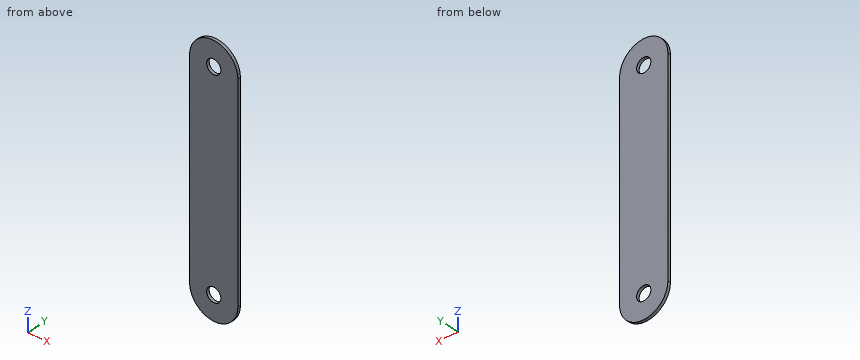
Solid Edge part; units mm, degrees
sketch "Sketch1" plane through (0, 0, 0) normal (0, -1, 0) x (1, 0, 0)
  circle A0 centre (0, 36.395) radius 2.5
  line L0 (-8.5, -36.755) -> (-8.5, 36.395)
  line L1 (8.5, 36.395) -> (8.5, -36.755)
  arc A1 (-8.5, 36.395) -> (8.5, 36.395) centre (0, 36.395) cw
  arc A2 (8.5, -36.755) -> (-8.5, -36.755) centre (0, -36.755) cw
  circle A3 centre (0, -36.755) radius 2.5
extrude "Protrusion1" add sketch "Sketch1" along normal blind 1
Geometry check sheet. Reference: the model listing, model coordinates, mm. Coordinates: 2 decimals unless noted, no trailing zeros. Order: outer loops, then holes, each group sorted by start corner. A loop starts at its lowest first (then second) coordinate and runs counter-clockwise, first axis right, second up.
Q1. Sectioned sample at C-C on x = 7.25. Record the cut outline in (y, z), and give its area (3 significant figures).
Reply:
outline: (-1, -41.19) - (0, -41.19) - (0, 40.83) - (-1, 40.83) - close
area: 82.0 mm2
Q2. Thickness scan on probe 1 along Z at (x, y) = (0, -0.45) (3 decimals); probe 2 along Z at (x, y) = (-2, -0.35) (3 decimals); probe 3 along X at (y, z) = (-0.6, -38.5). Record the ranges inside material, lowest first.
Reply:
probe 1: z = -45.255 to -39.255, -34.255 to 33.895, 38.895 to 44.895
probe 2: z = -45.016 to -38.255, -35.255 to 34.895, 37.895 to 44.656
probe 3: x = -8.32 to -1.79, 1.79 to 8.32
Q3. Sectioned sample at D-D on x = -6. Record the cut outline in (y, z), and give its area (3 significant figures).
Reply:
outline: (-1, -42.78) - (0, -42.78) - (0, 42.42) - (-1, 42.42) - close
area: 85.2 mm2
Q4. Sectioned sample at A-A on x = 0. Record the cut outline in (y, z) (3 decimals), and give its area (4 significant figures).
Reply:
outline: (-1, -45.255) - (0, -45.255) - (0, -39.255) - (-1, -39.255) - close; (-1, -34.255) - (0, -34.255) - (0, 33.895) - (-1, 33.895) - close; (-1, 38.895) - (0, 38.895) - (0, 44.895) - (-1, 44.895) - close
area: 80.15 mm2
Q5. Sectioned sample at B-B on y = -0.25. Record the cut outline in (x, z) (3 decimals), and give its area (3 significant figures).
Reply:
outline: (-8.5, -36.755) arc R8.5 ccw to (8.5, -36.755) - (8.5, 36.395) arc R8.5 ccw to (-8.5, 36.395) - close; hole circle Ø5 at (0, -36.755); hole circle Ø5 at (0, 36.395)
area: 1,430 mm2
